Verification items for the finished model (mm, model axes). Face numbers are marked on the shaded views. Give positions to 0.01 mm unless a question says otherwise; leave off trailing zeros. Write each loop counter-clockwise with the first axis right and the second up, starting at its lowest first coordinate (ties: lowest second). Pieces come first, ordered by that corner, then holes. Notation, with made-up numbers: (29.25, -10.5) -> (57.25, -10.5) arc R24 ccw to (57.25, 23.5) -> close; hole circle Ø10 at (31, 31.25). An arc over 180 degrees is marked (long way). Answer as CSV lines item,"result". Start each with the question number.
1) Material ranges on L1, parallel to X at y = 4, z = 0; L2, parallel to Z at x = 16.5, y = 1.7; L3, parallel to X at y = 4.55, z = 53, recorded low to high.
2) Sectioned sample at C-C on x = -52. Record the cut outline in (y, z), and give its area (3 significant figures).
3) Mould release check, pull along Z, two halves, no side actions. Record for the marked faces 1 and 2: released by +Z, released by -Z, zero draft, split by the parting line, or undercut.
4) Sectioned sample at D-D on y = 4.4. Record the cut outline in (x, z), and give its area (3 significant figures).
5) Gauge pin test, flat ends, axial feed: pin 1 Ø1 at (x, z) = (10, 49.5) entering from +Y; pin 2 Ø2 at (y, z) = (1.5, 37) entering from -X; pin 3 Ø1.5 at (x, y) = (30.5, 1) entering from -Z. Record the tip position at first contact, or that the pin passes through.
```python
from build123d import *

# Parameters (mm, degrees)
SMUSSO1_SIZE = 3


with BuildPart() as part:
    # Schizzo1 → Rivoluzione1 (revolve)
    with BuildSketch(Plane.XY, mode=Mode.PRIVATE) as rivoluzione1_sk:
        Polygon((-25.5, 0), (-25.5, 3), (-71, 3), (-71, 6), (-72, 6), (-72, 3), (-73, 3), (-73, 0), align=None)
    revolve(rivoluzione1_sk.sketch.rotate(Axis((0, 0, 0), (0, 1, 0)), 270), axis=Axis((0, 0, 0), (0, 1, 0)))

    # Smusso1
    smusso1_edges = [part.edges().sort_by_distance(p)[0] for p in [
        (0, 3, 25.5),
    ]]
    chamfer(smusso1_edges, length=SMUSSO1_SIZE - 0.0001)  # a hair under: the kernel refuses the full size


solid = part.part
```
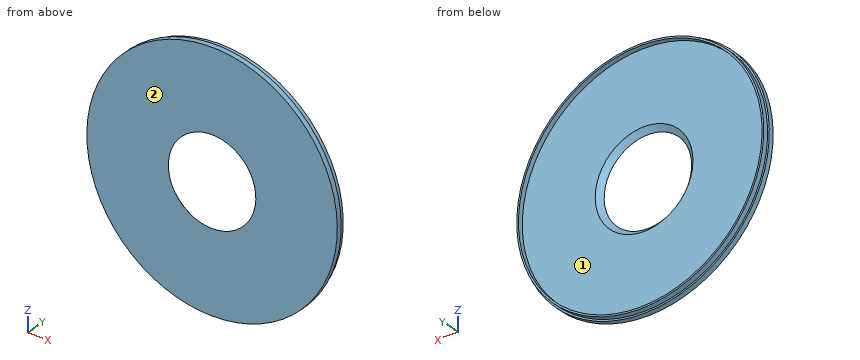
Ans:
1,L1,"x = -72 to -71, 71 to 72"
1,L2,"z = -71.11 to -21.62, 21.62 to 71.11"
1,L3,"x = -48.73 to -47.24, 47.24 to 48.73"
2,outline,"(0, -51.23) -> (3, -51.23) -> (3, -49.8) -> (6, -49.8) -> (6, -48.34) -> (3, -48.34) -> (3, 48.34) -> (6, 48.34) -> (6, 49.8) -> (3, 49.8) -> (3, 51.23) -> (0, 51.23) -> close"
2,area,"316 mm²"
3,face 1,"undercut"
3,face 2,"zero draft"
4,outline,"circle Ø144 at (0, 0); hole circle Ø142 at (0, 0)"
4,area,"449 mm²"
5,pin 1,"stops at y = 3"
5,pin 2,"stops at x = -63.51"
5,pin 3,"stops at z = -66.66"
